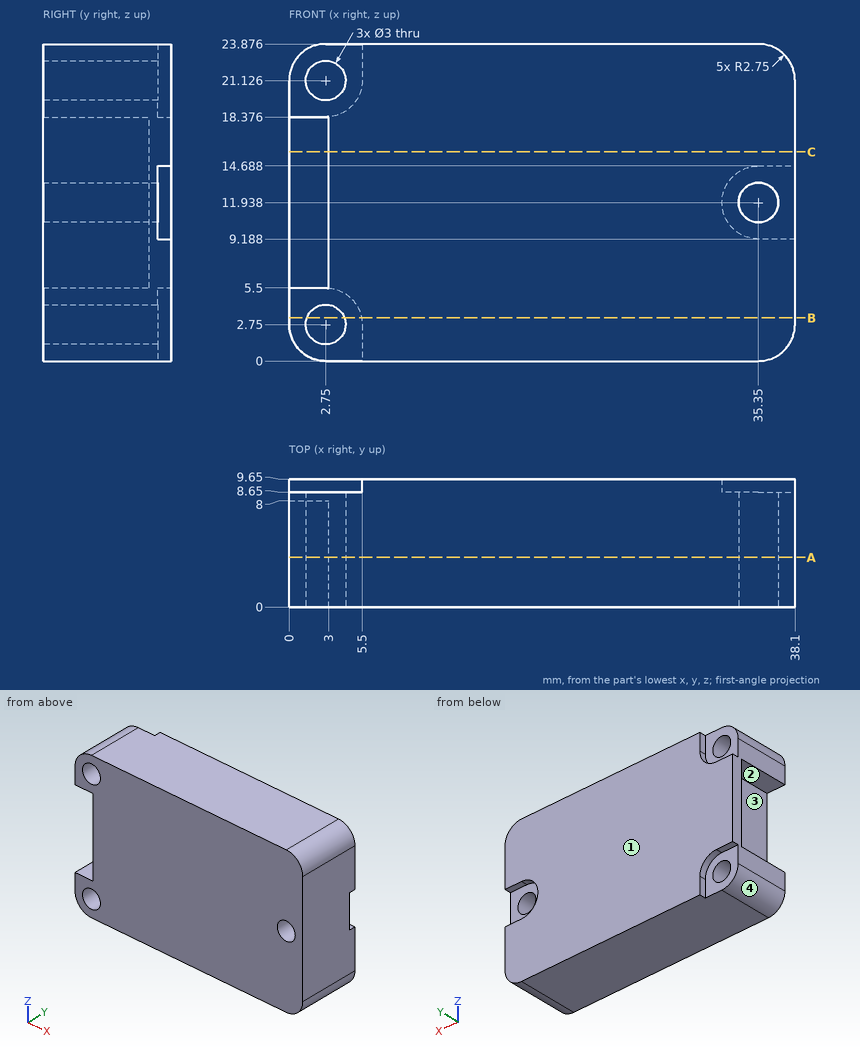
Here's the drawing with two shaded views (mm, measured from the low corner). I have some questions. Coordinates: 2 decimals unless noted, no trailing zeros. Write each loop counter-clockwise with the first axis right and the second up, starting at its lowest first coordinate (ties: lowest second). Pieces come first, ordered by that corner, then holes.
Item 1: I want a section at A-A on y = 3.75. Write out the boundary of the cut face in (x, z), and give its area (3 significant figures).
Item 2: If I drill on line 1 (X direction, y = 4.5, z = 6); line 2 (X direction, y = 7, z = 11.5); line 3 (X direction, y = 5, z = 19.75), over which ranges is the centre line in solid material (lowest first)?
Item 3: If we mould it in two halves opening along Z, with no side actions, what happens to the marked faces 1, 2, 3 and 4? For each: +Z half, -Z half, draft (parallel to the pull), parting line (faces both ways), or undercut.
Item 4: I want a section at C-C on z = 15.75. Write out the boundary of the cut face in (x, y), and give its area (3 significant figures).
Item 5: Will these pins go through, and if not, where does the flat tip stop? pin 1 (4 mm diameter, centred on y = 2, z = 14, fed in from -X); pin 2 (1.1 mm diameter, centred on x = 37.5, y = 9, fed in from +Z); pin 3 (2.5 mm diameter, centred on x = 1, z = 12, fed in from -Y).
Item 6: I want a section at B-B on z = 3.25. Write out the boundary of the cut face in (x, y).
Findings below:
1. outline: (0, 2.75) arc R2.75 ccw to (2.75, 0) - (35.35, 0) arc R2.75 ccw to (38.1, 2.75) - (38.1, 21.13) arc R2.75 ccw to (35.35, 23.88) - (2.75, 23.88) arc R2.75 ccw to (0, 21.13) - (0, 18.38) - (3, 18.38) - (3, 5.5) - (0, 5.5) - close; hole circle Ø3 at (2.75, 2.75); hole circle Ø3 at (2.75, 21.13); hole circle Ø3 at (35.35, 11.94)
1. area: 843 mm2
2. line 1: x = 3 to 38.1
2. line 2: x = 3 to 33.92, 36.78 to 38.1
2. line 3: x = 0 to 2.15, 3.35 to 38.1
3. face 1: draft
3. face 2: undercut
3. face 3: undercut
3. face 4: -Z half
4. outline: (0, 8) - (3, 8) - (3, 0) - (38.1, 0) - (38.1, 9.65) - (0, 9.65) - close
4. area: 344 mm2
5. pin 1: stops at x = 3
5. pin 2: stops at z = 23.36
5. pin 3: stops at y = 8
6. outline: (0, 0) - (1.34, 0) - (1.34, 8.65) - (0, 8.65) - close; (4.16, 0) - (38.1, 0) - (38.1, 9.65) - (5.45, 9.65) - (5.45, 8.65) - (4.16, 8.65) - close
